CAD build for the part. Positions are in the model's coordinates, mm. A direction names the side the tool comes from. Give positions to 0.01 mm unless a question says otherwise; leave off trailing zeros. Write each loop counter-clockwise with the first axis right and the second up, starting at its lowest first coordinate (ties: lowest second). Pieces come first, ordered by that corner, then holes. Notation, with made-up numbers: (38.25, -5.75) - (81.25, -5.75) arc R22 ccw to (81.25, 6.25) - close; hole circle Ø6 at (89, -24.75). An arc over 180 degrees is marked (long way). Answer as a JSON object with one key per item and string values.
from build123d import *

# Parameters (mm, degrees)
SKETCH_2_W               = 1.2
SKETCH_2_H               = 1.2
CUT_EXTRUDE_1_DEPTH      = 3
CUT_EXTRUDE_1_DEPTH_BACK = 3
CHAMFER_1_SIZE           = 0.4
FILLET_1_R               = 1
FILLET_2_R               = 0.4


with BuildPart() as part:
    # Эскиз1 → Повернуть1 (revolve)
    with BuildSketch(Plane(origin=(0, 0, 0), x_dir=(1, 0, 0), z_dir=(0, 1, 0))):
        Polygon((0, 0), (-2, 0), (-2, 1.8), (-1, 1.8), (-1, 23.25), (0, 23.25), align=None)
    revolve(axis=Axis((0, 0, -23.25), (0, 0, 1)))

    # Эскиз2 → Вырез-Вытянуть1 (cut, two sides)
    with BuildSketch(Plane(origin=(0, 0, 0), x_dir=(0, 0, -1), z_dir=(1, 0, 0))) as cut_extrude_1_sk:
        with Locations((0.6, 0)):
            Rectangle(SKETCH_2_W, SKETCH_2_H)
    extrude(amount=CUT_EXTRUDE_1_DEPTH, mode=Mode.SUBTRACT)
    extrude(cut_extrude_1_sk.sketch, amount=-CUT_EXTRUDE_1_DEPTH_BACK, mode=Mode.SUBTRACT)

    # Фаска1
    chamfer_1_edges = [part.edges().sort_by_distance(p)[0] for p in [
        (1, 0, -23.25),
    ]]
    chamfer(chamfer_1_edges, length=CHAMFER_1_SIZE)

    # Скругление1
    fillet_1_edges = [part.edges().sort_by_distance(p)[0] for p in [
        (0, 2, 0),
        (0, -2, 0),
    ]]
    fillet(fillet_1_edges, radius=FILLET_1_R)

    # Скругление2
    fillet_2_edges = [part.edges().sort_by_distance(p)[0] for p in [
        (1, 0, -1.8),
    ]]
    fillet(fillet_2_edges, radius=FILLET_2_R)


solid = part.part
(1) Pull direction Y, two halves, no side cores. Call faces 1 (the face through (0, 0, -1.2)), 2 (the face through (0, 1, -13)), 3 (the face through (0, 0, -23.25)): pulls with the +Y half, pulls with the -Y half, needs draft (parallel to the pull), parting line crosses it, or undercut.
Answer key:
{"face 1": "undercut", "face 2": "parting line crosses it", "face 3": "needs draft"}
(2) Probe L1, parallel to Y at x = 0.8, z = -6.5; L2, parallel to Z at x = 0.3, y = -0.5; L3, parallel to Y at x = -0.6, z = -8. List the from-to ranges inside material, lowest first. Write a range as [from, to].
Answer key:
{"L1": "y = [-0.6, 0.6]", "L2": "z = [-23.25, -1.2]", "L3": "y = [-0.8, 0.8]"}
(3) Flat gauge pins, fed straight in: P1, Ø1, axis at x = 1, z = -0.5, coming from the -Y side; P2, Ø1.2, axis at x = 0.5, y = -0.5, coming from the -Z side; P3, Ø0.6, axis at x = 0.5, y = 0, coming from the +Z side. Where does each tip first touch, or does it go through?
Answer key:
{"P1": "stops at y = -1.89", "P2": "stops at z = -23.25", "P3": "stops at z = -1.2"}
(4) 3-axis set-ups, long thin cutter, end or side, ignore diameter. For faces 4 (the face through (-1.847, 0.766, -1.406)), 5 (the face through (0, -0.6, -1)), 6 (the face through (-0.9, 1.3, -1.8)): which of +Z, -Z, +X, -X, +Y, -Y reach the whole face in a straight line?
Answer key:
{"face 4": "+Z, -Z", "face 5": "+Z, +X, -X", "face 6": "-Z"}
(5) Saw through at A-A, the plane z = -17.5. Give the cut face in (x, y), and give its area (3 significant figures).
Answer key:
{"outline": "circle Ø2 at (0, 0)", "area": "3.14 mm²"}
